The listing builds one solid part. Answer for the finished solid, in the listing's coordinates (mm). Face numbers are marked on the shaded views. A direction names the side the tool comes from. Round coordinates to 2 decimals unless told otherwise and drop trailing zeros. Order: outer loops, then holes, each group sorted by start corner. A loop starts at its lowest first (then second) coordinate and runs counter-clockwise, first axis right, second up. Notation, with made-up numbers: M 72.25,70 L 80.25,70 A27 cw 80.25,97 Z; hole C 69,22.5 d8. An arc over 180 degrees is marked long. Put each result on its own line as item: value. Start each with the question number.
1. The part is cut by section A-A (y = -6). Give the vertices of the cut face in (x, z).
2. The part is cut by section B-B (x = -47). Give the vertices of the cut face in (y, z), then the cut area to 3 significant figures.
3. The part is cut by section D-D (x = -22.5). Give the vertices of the cut face in (y, z).
4. Each of these flat-tipped pins is pushed along its axis until it touches: pin 1 Ø3 at (x, z) = (2.5, 5.5) entering from -Y; pin 2 Ø2 at (x, z) = (-21.5, 3.5) entering from -Y; pin 3 Ø2 at (x, z) = (-40.5, 3) entering from -Y. Where does it stop, or does it pass through?
5. Consider line 1 (X direction, y = 2, z = -6); line 2 (X direction, y = -26, z = -0.75); line 3 (Y direction, x = 9, z = 3.5). Determine where each line is inside the solid, lowest interval first.
6. The part is cut by section C-C (y = 4.5). Give the vertices of the cut face in (x, z), then the cut area to 3 significant figures.
7. Which of the six approach directions +Z, -Z, +X, -X, +Y, -Y give full straight-line access (tool end or side, diameter ignored) to the marked faces 3, 4, 5 and 6?
8. The mould has two halves that part along X. Classify the marked faces 1 and 2: +X half, -X half, draft (parallel to the pull), parting line (faces both ways), or undercut.
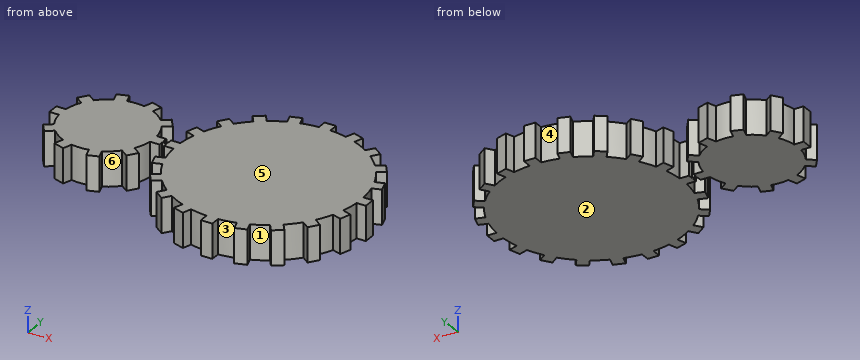
from build123d import *

# Parameters (mm, degrees)
SKETCH_2_R               = 20
EXTRUDE_2_DEPTH          = 15
SKETCH_7_R               = 40
EXTRUDE_4_DEPTH          = 15
SKETCH_9_W               = 5
SKETCH_9_H               = 5
EXTRUDE_6_DEPTH          = 15
PATTERN_CIRCULAR_1_COUNT = 10
SKETCH_17_W              = 5
SKETCH_17_H              = 5
EXTRUDE_9_DEPTH          = 15
PATTERN_CIRCULAR_3_COUNT = 20
SKETCH_18_W              = 3
SKETCH_18_H              = 1
EXTRUDE_10_DEPTH         = 15


with BuildPart() as part:
    # Sketch 2 → Extrude 2 (new body)
    with BuildSketch(Plane.XY.offset(-7.5)):
        with Locations((-35, 0)):
            Circle(SKETCH_2_R)
    extrude(amount=EXTRUDE_2_DEPTH)

    # Sketch 9 → Extrude 6 (add)
    with BuildSketch(Plane.XY.offset(-7.5)):
        with Locations((-13.5, 0)):
            Rectangle(SKETCH_9_W, SKETCH_9_H)
    extrude_6 = extrude(amount=EXTRUDE_6_DEPTH)

    # Pattern Circular 1: Extrude 6 ×10 about axis
    pattern_circular_1_axis = Axis((-35, 0, 0), (0, 0, 1))
    for i in range(1, PATTERN_CIRCULAR_1_COUNT):
        add(extrude_6.rotate(pattern_circular_1_axis, i * 360 / PATTERN_CIRCULAR_1_COUNT))



with BuildPart() as body_2:
    # Sketch 7 → Extrude 4 (new body)
    with BuildSketch(Plane.XY.offset(-7.5)):
        with Locations((35, 0)):
            Circle(SKETCH_7_R)
    extrude(amount=EXTRUDE_4_DEPTH)

    # Sketch 17 → Extrude 9 (add)
    with BuildSketch(Plane.XY.offset(-7.5)):
        with Locations((-6.5, 0)):
            Rectangle(SKETCH_17_W, SKETCH_17_H)
    extrude_9 = extrude(amount=EXTRUDE_9_DEPTH)

    # Pattern Circular 3: Extrude 9 ×20 about axis
    pattern_circular_3_axis = Axis((35, 0, 0), (0, 0, 1))
    for i in range(1, PATTERN_CIRCULAR_3_COUNT):
        add(extrude_9.rotate(pattern_circular_3_axis, i * 360 / PATTERN_CIRCULAR_3_COUNT))


with BuildPart() as part_1:
    add(part.part)

    add(body_2.part)  # Extrude 10 merges body 2
    # Sketch 18 → Extrude 10 (add)
    with BuildSketch(Plane.XY.offset(-7.5)):
        with Locations((-10, 0)):
            Rectangle(SKETCH_18_W, SKETCH_18_H)
    extrude(amount=EXTRUDE_10_DEPTH)


solid = part_1.part
Resolved:
1. outline: M -54.08,-7.5 L -15.92,-7.5 L -15.92,7.5 L -54.08,7.5 Z; M -4.55,-7.5 L 74.55,-7.5 L 74.55,7.5 L -4.55,7.5 Z
2. outline: M -16,-7.5 L 16,-7.5 L 16,7.5 L -16,7.5 Z
2. area: 480 mm2
3. outline: M -15.61,-7.5 L 15.61,-7.5 L 15.61,7.5 L -15.61,7.5 Z
4. pin 1: y = -27.79
4. pin 2: y = -15.61
4. pin 3: y = -23.6
5. line 1: -59 to -11, -9 to 79
5. line 2: -0.5 to 3.47, 4.6 to 65.4, 66.53 to 70.5
5. line 3: -35.5 to -31.53, -30.4 to 30.4, 31.53 to 35.5
6. outline: M -54.49,-7.5 L -15.51,-7.5 L -15.51,7.5 L -54.49,7.5 Z; M -4.75,-7.5 L 74.75,-7.5 L 74.75,7.5 L -4.75,7.5 Z
6. area: 1,780 mm2
7. face 3: +Z, -Z, -Y
7. face 4: +Z, -Z, +Y
7. face 5: +Z, +X, -X, +Y, -Y
7. face 6: +Z, -Z
8. face 1: undercut
8. face 2: draft
